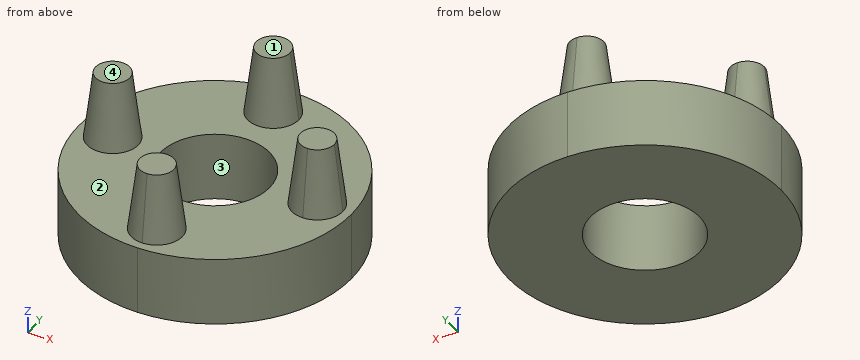
```python
from build123d import *

# Parameters (mm, degrees)
F0_R     = 4
F1_DEPTH = 5
F3_R     = 1.25
F6_COUNT = 4


# Not quite as in the source:
# - a feature names something its author has since deleted; it is built from what else it names


with BuildPart() as f1:
    # F0 (on Top) → F1 (new body)
    with BuildSketch(Plane.XY):
        with BuildLine():
            ThreePointArc((0, 10), (-7.0710678119, -7.0710678119), (10, 0))
            ThreePointArc((10, 0), (7.0710678119, 7.0710678119), (0, 10))
        make_face()
        Circle(F0_R, mode=Mode.SUBTRACT)
        with BuildLine():
            ThreePointArc((2.5, 7.5), (-1.767766953, 5.732233047), (0, 10))
            ThreePointArc((0, 10), (1.767766953, 9.267766953), (2.5, 7.5))
        make_face(mode=Mode.SUBTRACT)
        with BuildLine():
            ThreePointArc((2.5, 7.5), (1.767766953, 9.267766953), (0, 10))
            ThreePointArc((0, 10), (-1.767766953, 5.732233047), (2.5, 7.5))
        make_face()
    extrude(amount=F1_DEPTH)

    # F3 (on offset) → F4 section 0
    with BuildSketch(Plane.XY.offset(10)):
        with Locations((0, 7.5)):
            Circle(F3_R)
    # F0 (on Top) → F4 section 1
    with BuildSketch(Plane.XY):
        with BuildLine():
            ThreePointArc((2.5, 7.5), (1.767766953, 9.267766953), (0, 10))
            ThreePointArc((0, 10), (-1.767766953, 5.732233047), (2.5, 7.5))
        make_face()
    loft()

    # F6: F1 ×4 about axis
    f6_axis = Axis((0, 0, 16.9871691614), (0, 0, 1))


with BuildPart() as f1_1:
    add(f1.part)
    for i in range(1, F6_COUNT):
        add(f1.part.rotate(f6_axis, i * 360 / F6_COUNT))


solid = f1_1.part
```
Check sheet for the modelled part. Datum: model origin and axes. Units: mm. Face numbers are marked on the shaded views. A direction names the side the tool comes from. Coordinates: 2 decimals unless noted, no trailing zeros. Write each loop counter-clockwise with the first axis right and the second up, starting at its lowest first coordinate (ties: lowest second). Pieces come first, ordered by that corner, then holes. Notation, with made-up numbers: (57.5, -28.75) -> (66.5, -28.75) arc R10 ccw to (66.5, -21.75) -> close; hole circle Ø9 at (80.25, 31). An arc over 180 degrees is marked (long way). Use a Markdown table: item, result.
1. Sectioned sample at A-A (z = 9). Enter the section's corners in (x, y) (3 decimals).
Reported:
| item | result |
|---|---|
| outline | circle Ø2.75 at (-7.5, 0); circle Ø2.75 at (0, -7.5); circle Ø2.75 at (0, 7.5); circle Ø2.75 at (7.5, 0) |
2. Sectioned sample at B-B (x = 3.75). Enter the section's corners in (y, z).
Reported:
| item | result |
|---|---|
| outline | (-9.27, 0) -> (-1.39, 0) -> (-1.39, 5) -> (-9.27, 5) -> close; (1.39, 0) -> (9.27, 0) -> (9.27, 5) -> (1.39, 5) -> close |
3. Tool access check on the marked faces 1 and 2. Record the directions out of +Z, -Z, +X, -X, +Y, -Y that give a thin tool (end or side, any length) a straight path to the whole face; none if there is none.
Reported:
| item | result |
|---|---|
| face 1 | +Z, +X, -X, +Y, -Y |
| face 2 | +Z |
4. Sectioned sample at C-C (z = 2). Enter the section's corners in (x, y), plus the area to 3 significant figures.
Reported:
| item | result |
|---|---|
| outline | circle Ø20 at (0, 0); hole circle Ø8 at (0, 0) |
| area | 264 mm2 |
5. Release check for a two-part mould opening along X. For the marked faces 3 and 4 record: pulls with the +X half, pulls with the -X half, needs draft (parallel to the pull), parting line crosses it, or undercut.
Reported:
| item | result |
|---|---|
| face 3 | undercut |
| face 4 | needs draft |
6. Sectioned sample at D-D (x = -2.5). Enter the section's corners in (y, z), plus the area to 3 significant figures.
Reported:
| item | result |
|---|---|
| outline | (-9.68, 0) -> (-3.12, 0) -> (-3.12, 5) -> (-9.68, 5) -> close; (3.12, 0) -> (9.68, 0) -> (9.68, 5) -> (3.12, 5) -> close |
| area | 65.6 mm2 |
7. Scan lines: line 1 along Y through (x, z) = (0, 1.9); line 2 along Z through (x, y) = (-4.5, -6); line 3 along Y through (x, z) = (-1, 4). Record each from-to range of solid material in increasing order.
Reported:
| item | result |
|---|---|
| line 1 | y = -10 to -4, 4 to 10 |
| line 2 | z = 0 to 5 |
| line 3 | y = -9.95 to -3.87, 3.87 to 9.95 |
8. Go/stop test with flat-tipped pins: pin 1 Ø5 at (x, z) = (5, 8.5) entering from +Y; pin 2 Ø3 at (x, z) = (-4, 7.5) entering from -Y; pin 3 Ø4 at (x, z) = (-5.5, 4) entering from +Y; pin 4 Ø3 at (y, z) = (-6.5, 3) entering from +X. Record where each tip stops, or that it passes through.
Reported:
| item | result |
|---|---|
| pin 1 | stops at y = 1.56 |
| pin 2 | passes through |
| pin 3 | stops at y = 9.37 |
| pin 4 | stops at x = 8.66 |
